from build123d import *

# Parameters (mm, degrees)
SKETCH1_R                = 60.394691442
BOSS_EXTRUDE1_DEPTH      = 1
BOSS_EXTRUDE3_START      = 4
SKETCH3_R                = 9
BOSS_EXTRUDE3_DEPTH      = 14
CUT_EXTRUDE1_START       = 6
SKETCH4_R                = 1.3
CUT_EXTRUDE1_DEPTH       = 99.311500824
BOSS_EXTRUDE4_DEPTH      = 9
BOSS_EXTRUDE4_DEPTH_BACK = 14
CUT_EXTRUDE2_DEPTH       = 108.867849616
CUT_EXTRUDE2_DEPTH_BACK  = 108.867849616
FILLET1_R                = 10
FILLET3_R                = 2
BOSS_EXTRUDE9_START      = 3
SKETCH11_R               = 60.394691442
SKETCH11_R_2             = 56.5
BOSS_EXTRUDE9_DEPTH      = 3
SKETCH14_R               = 46.5
SKETCH14_W               = 15
SKETCH14_H               = 30
BOSS_EXTRUDE12_DEPTH     = 3
SKETCH16_R               = 2
CUT_EXTRUDE3_DEPTH       = 4


with BuildPart() as part:
    # Sketch1 → Boss-Extrude1 (new body)
    with BuildSketch(Plane(origin=(0, 0, 0), x_dir=(1, 0, 0), z_dir=(0, 1, 0))):
        with Locations(Location((0, 0, 0), (0, 0, 270))):
            Circle(SKETCH1_R)
    extrude(amount=BOSS_EXTRUDE1_DEPTH)

    # Sketch3 → Boss-Extrude3 (add)
    with BuildSketch(Plane(origin=(0, 0, 0), x_dir=(0, 0, -1), z_dir=(1, 0, 0)).offset(BOSS_EXTRUDE3_START)):
        with BuildLine():
            Line((-30.34, 1), (30.34, 1))
            Line((30.34, 1), (30.34, 8.64))
            ThreePointArc((30.34, 8.64), (31.482215556, 14.381237698), (34.73490804, 19.248111261))
            ThreePointArc((34.73490804, 19.248111261), (35.146816919, 52.490993137), (1.923997232, 53.717009602))
            Line((1.923997232, 53.717009602), (-18.767804398, 34.964811646))
            ThreePointArc((-18.767804398, 34.964811646), (-27.317276732, 23.137402619), (-30.34, 8.86))
            Line((-30.34, 8.86), (-30.34, 1))
        make_face()
        with Locations(Location((17.907195719, 36.080614483, 0), (0, 0, 180))):
            Circle(SKETCH3_R, mode=Mode.SUBTRACT)
    extrude(amount=BOSS_EXTRUDE3_DEPTH)

    # Sketch4 → Cut-Extrude1 (cut, through all)
    with BuildSketch(Plane(origin=(0, 0, 0), x_dir=(0, 0, -1), z_dir=(1, 0, 0)).offset(CUT_EXTRUDE1_START)):
        with Locations(Location((23.599251188, 50.305537875, 0), (0, 0, 180))):
            Circle(SKETCH4_R)
        with Locations(Location((31.162882913, 43.764018545, 0), (0, 0, 180))):
            Circle(SKETCH4_R)
        with Locations(Location((-0.236409868, 7.458586268, 0), (0, 0, 180))):
            Circle(SKETCH4_R)
        with Locations(Location((-7.800041592, 14.000105597, 0), (0, 0, 180))):
            Circle(SKETCH4_R)
        Polygon((17.149721975, 51.256102402), (33.033348596, 37.518911811), (6.213119346, 6.50802174), (-9.670507276, 20.245212332), align=None)
    extrude(amount=CUT_EXTRUDE1_DEPTH, mode=Mode.SUBTRACT)

    # Sketch8 → Boss-Extrude4 (add, two sides: drawn at the far end of the back side and taken through both)
    with BuildSketch(Plane(origin=(18, 0, 0), x_dir=(0, 0, -1), z_dir=(1, 0, 0)).offset(-BOSS_EXTRUDE4_DEPTH_BACK)):
        with BuildLine():
            Line((-30.34, 1), (-30.34, 8.86))
            ThreePointArc((-30.34, 8.86), (-27.317276732, 23.137402619), (-18.767804398, 34.964811646))
            Line((-18.767804398, 34.964811646), (1.923997232, 53.717009602))
            ThreePointArc((1.923997232, 53.717009602), (35.146816919, 52.490993137), (34.73490804, 19.248111261))
            ThreePointArc((34.73490804, 19.248111261), (31.482215556, 14.381237698), (30.34, 8.64))
            Line((30.34, 8.64), (30.34, 1))
            Line((30.34, 1), (36.34, 1))
            Line((36.34, 1), (36.34, 8.64))
            ThreePointArc((36.34, 8.64), (37.025329334, 12.084742619), (38.976944824, 15.004866757))
            ThreePointArc((38.976944824, 15.004866757), (39.492690314, 56.627825795), (-2.105149131, 58.162904291))
            Line((-2.105149131, 58.162904291), (-22.796950761, 39.410706335))
            ThreePointArc((-22.796950761, 39.410706335), (-32.802478559, 25.568978426), (-36.34, 8.86))
            Line((-36.34, 8.86), (-36.34, 1))
            Line((-36.34, 1), (-30.34, 1))
        make_face()
    extrude(amount=BOSS_EXTRUDE4_DEPTH + BOSS_EXTRUDE4_DEPTH_BACK)

    # Sketch10 → Cut-Extrude2 (cut, two sides: drawn at the far end of the back side and taken through both)
    with BuildSketch(Plane.XY.offset(-CUT_EXTRUDE2_DEPTH_BACK)):
        with BuildLine():
            Line((27, 65.881981391), (21, 65.881981391))
            ThreePointArc((21, 65.881981391), (22.692685718, 33.351362906), (26.5, 1))
            Line((26.5, 1), (27, 1))
            Line((27, 1), (27, 65.881981391))
        make_face()
    extrude(amount=CUT_EXTRUDE2_DEPTH + CUT_EXTRUDE2_DEPTH_BACK, mode=Mode.SUBTRACT)

    # Fillet1
    fillet1_edges = [part.edges().sort_by_distance(p)[0] for p in [
        (4, 12.084742619, -37.025329334),
        (4, 25.568978426, 32.802478559),
        (4, 4.93, 36.34),
        (4, 4.82, -36.34),
        (4, 56.627825795, -39.492690314),
        (4, 48.786805313, 12.451049946),
    ]]
    fillet(fillet1_edges, radius=FILLET1_R)

    # Fillet3
    fillet3_edges = [part.edges().sort_by_distance(p)[0] for p in [
        (20.25, 1, -36.34),
        (6.928932188, 1, -33.411067812),
        (4, 1, 0),
        (6.928932188, 1, 33.411067812),
        (20.25, 1, 36.34),
    ]]
    fillet(fillet3_edges, radius=FILLET3_R)
    fillet3_2_edges = [part.edges().sort_by_distance(p)[0] for p in [
        (26.5, 1, -33.34),
    ]]
    fillet(fillet3_2_edges, radius=FILLET3_R)
    fillet3_3_edges = [part.edges().sort_by_distance(p)[0] for p in [
        (26.5, 1, 33.34),
    ]]
    fillet(fillet3_3_edges, radius=FILLET3_R)

    # Sketch11 → Boss-Extrude9 (add)
    with BuildSketch(Plane.XZ.offset(BOSS_EXTRUDE9_START)):
        with Locations(Location((0, 0, 0), (0, 0, 270))):
            Circle(SKETCH11_R)
        with Locations(Location((0, 0, 0), (0, 0, 270))):
            Circle(SKETCH11_R_2, mode=Mode.SUBTRACT)
    extrude(amount=-BOSS_EXTRUDE9_DEPTH)

    # Sketch14 → Boss-Extrude12 (add)
    with BuildSketch(Plane(origin=(0, 0, 0), x_dir=(-1, 0, 0), z_dir=(0, -1, 0))):
        with Locations(Location((0, 0, 0), (0, 0, 270))):
            Circle(SKETCH14_R)
        Rectangle(SKETCH14_W, SKETCH14_H, mode=Mode.SUBTRACT)
    extrude(amount=BOSS_EXTRUDE12_DEPTH)

    # Sketch16 → Cut-Extrude3 (cut)
    with BuildSketch(Plane(origin=(0, 0, 0), x_dir=(-1, 0, 0), z_dir=(0, -1, 0))):
        with Locations(Location((5.032683159, 10, 0), (0, 0, 90))):
            Circle(SKETCH16_R)
        with Locations(Location((5.032683159, -10, 0), (0, 0, 90))):
            Circle(SKETCH16_R)
    extrude(amount=-CUT_EXTRUDE3_DEPTH, mode=Mode.SUBTRACT)


solid = part.part
Input: part model. Units: mm. Frame: model coordinates. A direction names the side the tool comes from. Coordinates: 2 decimals unless noted, no trailing zeros. Loops run counter-clockwise (first coordinate to the right, second up) from the corner with the lowest first, then second, coordinate; pieces in that order, holes last.
(1) Section A-A on x = 0. Return the cut outline in (y, z).
(2) Set-up query: faces 4 (the face through (-7.5, -1, 0)), 5 (the face through (4, 24, -5)), 6 (the face through (11.916, 44.484, -24.98)), 7 (the face through (20, 6, -36.34)). Return all of +Z, -Z, +X, -X, +Y, -Y with unobstructed straight access to the full face (end or side cutting, diameter ignored); none if empty.
(3) First-contact query: pin 1 Ø13 at (y, z) = (35, -18) entering from +X; pin 2 Ø10 at (y, z) = (17.5, 11.5) entering from -X; pin 3 Ø5 at (y, z) = (40, -8) entering from +X; pin 4 Ø1.3 at (y, z) = (44, -31) entering from +X. Flat tips, straight axial feed; report the tip coordinate or a pass-through.
(4) Section C-C on x = -19.5. Return the cut outline in (y, z).
(5) Material intervals for probe 1 along X at (y, z) = (-1, 0); probe 2 along Z at (x, y) = (18.5, 5.5); probe 3 along Y at (x, z) = (48, 33), sorted ascending.
(6) Section B-B on x = -42. Return the cut outline in (y, z), then the cut area to 3 significant figures.
(7) Pull-direction query (Y, two-part tool) for faces 1 (the face through (22, 5, -30.34)), 2 (the face through (18.3, 25.8, 32.7)), 3 (the face through (-46.1, -1.5, -6.1)); classes: released by +Y, released by -Y, zero draft, split by the parting line, or undercut.
Data:
1. outline: (-3, -60.39) - (1, -60.39) - (1, 60.39) - (-3, 60.39) - (-3, 56.5) - (0, 56.5) - (0, 46.5) - (-3, 46.5) - (-3, 15) - (0, 15) - (0, -15) - (-3, -15) - (-3, -46.5) - (0, -46.5) - (0, -56.5) - (-3, -56.5) - close
2. face 4: -Y
2. face 5: +Z, -Z, -X, +Y
2. face 6: +X
2. face 7: -Z, +X, -X
3. pin 1: passes through
3. pin 2: stops at x = 4
3. pin 3: stops at x = 18
3. pin 4: stops at x = 6
4. outline: (-3, -57.16) - (1, -57.16) - (1, 57.16) - (-3, 57.16) - (-3, 53.03) - (0, 53.03) - (0, 42.21) - (-3, 42.21) - (-3, -42.21) - (0, -42.21) - (0, -53.03) - (-3, -53.03) - close
5. probe 1: x = -60.39 to -56.5, -46.5 to -7.5, 7.5 to 46.5, 56.5 to 60.39
5. probe 2: z = -36.34 to -30.34, 30.34 to 36.34
5. probe 3: y = -3 to 1
6. outline: (-3, -43.4) - (1, -43.4) - (1, 43.4) - (-3, 43.4) - (-3, 37.79) - (0, 37.79) - (0, 19.96) - (-3, 19.96) - (-3, -19.96) - (0, -19.96) - (0, -37.79) - (-3, -37.79) - close
6. area: 240 mm2
7. face 1: undercut
7. face 2: released by +Y
7. face 3: zero draft
